Model file for the job. Use its own axes, mm. Face numbers are marked on the shaded views. A direction names the side the tool comes from. Round coordinates to 2 decimals unless told otherwise and drop trailing zeros. Order: outer loops, then holes, each group sorted by start corner. A loop starts at its lowest first (then second) coordinate and runs counter-clockwise, first axis right, second up. Notation, with made-up numbers: M -12,35 L 22,35 A21 cw 22,63 Z; hole C 78.5,23.5 d1. An arc over 180 degrees is marked long. Return JSON: item names as keys, results as strings. Group by question number.
Item 1: Slice it at B-B on y = 0. Write the cut outline in (x, z), then the cut area to 3 significant figures.
Item 2: Which spindle directions (+Z, -Z, +X, -X, +Y, -Y) get a long thin tool onto all of the face, cutting with end or side? Do the marked faces 5 and 6. Say none if no direction does.
Item 3: Slice it at C-C on z = -0.5. Write the cut outline in (x, y).
Item 4: Slice it at D-D on y = 2. Write the cut outline in (x, z), then the cut area to 3 significant figures.
Item 5: Pull direction X, two halves, no side cores. Call the marked faces 1, 2, 3 and 4: pulls with the +X half, pulls with the -X half, needs draft (parallel to the pull), parting line crosses it, or undercut.
Item 6: Slice it at A-A on x = 0. Write the cut outline in (y, z).
Item 7: Pin check, flat tips, straight feed: pin 1 Ø5 at (x, z) = (0, -3) entering from -Y; pin 2 Ø5 at (x, z) = (0, 12) entering from +Y; pin 3 Ø6 at (y, z) = (2, 11.5) entering from -X. Stop position of each tip, or through.
Item 8: Probe line 1 along Z through (x, y) = (0, 2.25); line 2 along X through (y, z) = (-3.25, -3); line 3 along X through (y, z) = (0.75, -3). List the from-to ranges inside material, lowest first.
from build123d import *

# Parameters (mm, degrees)
SKETCH1_R               = 5.5
BOSS_EXTRUDE1_DEPTH     = 9
SKETCH2_R               = 4.5
BOSS_EXTRUDE2_DEPTH     = 6
SKETCH3_R               = 4.5
BOSS_EXTRUDE3_DEPTH     = 6
SKETCH4_R               = 1.5
CUT_EXTRUDE1_DEPTH      = 6.5
CUT_EXTRUDE1_DEPTH_BACK = 6.5


with BuildPart() as part:
    # Sketch1 → Boss-Extrude1 (new body)
    with BuildSketch(Plane.XY):
        Circle(SKETCH1_R)
    extrude(amount=BOSS_EXTRUDE1_DEPTH)

    # Sketch2 → Boss-Extrude2 (add)
    with BuildSketch(Plane.XY.offset(9)):
        Circle(SKETCH2_R)
    extrude(amount=BOSS_EXTRUDE2_DEPTH)

    # Sketch3 → Boss-Extrude3 (add)
    with BuildSketch(Plane(origin=(0, 0, 0), x_dir=(-1, 0, 0), z_dir=(0, 0, -1))):
        Circle(SKETCH3_R)
    extrude(amount=BOSS_EXTRUDE3_DEPTH)

    # Sketch4 → Cut-Extrude1 (cut, two sides)
    with BuildSketch(Plane(origin=(0, 0, 0), x_dir=(1, 0, 0), z_dir=(0, 1, 0))) as cut_extrude1_sk:
        with Locations((0, 3)):
            Circle(SKETCH4_R)
        with Locations((0, -12)):
            Circle(SKETCH4_R)
    extrude(amount=CUT_EXTRUDE1_DEPTH, mode=Mode.SUBTRACT)
    extrude(cut_extrude1_sk.sketch, amount=-CUT_EXTRUDE1_DEPTH_BACK, mode=Mode.SUBTRACT)


solid = part.part
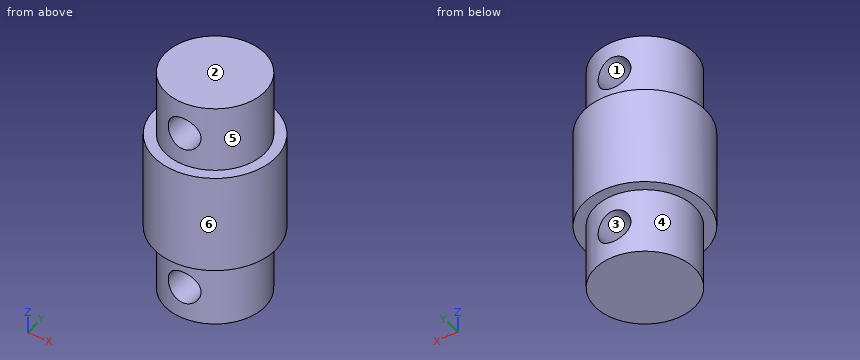
Output values:
{
 "1": {"outline": "M -5.5,0 L -4.5,0 L -4.5,-6 L 4.5,-6 L 4.5,0 L 5.5,0 L 5.5,9 L 4.5,9 L 4.5,15 L -4.5,15 L -4.5,9 L -5.5,9 Z; hole C 0,-3 d3; hole C 0,12 d3", "area": "193 mm²"},
 "2": {"face 5": "+Z", "face 6": "+Z, -Z"},
 "3": {"outline": "C 0,0 d9"},
 "4": {"outline": "M -5.12,0 L -4.03,0 L -4.03,-6 L 4.03,-6 L 4.03,0 L 5.12,0 L 5.12,9 L 4.03,9 L 4.03,15 L -4.03,15 L -4.03,9 L -5.12,9 Z; hole C 0,-3 d3; hole C 0,12 d3", "area": "175 mm²"},
 "5": {"face 1": "undercut", "face 2": "needs draft", "face 3": "undercut", "face 4": "parting line crosses it"},
 "6": {"outline": "M -5.5,0 L -4.5,0 L -4.5,-1.5 L 4.5,-1.5 L 4.5,0 L 5.5,0 L 5.5,9 L 4.5,9 L 4.5,10.5 L -4.5,10.5 L -4.5,9 L -5.5,9 Z; M -4.5,-6 L 4.5,-6 L 4.5,-4.5 L -4.5,-4.5 Z; M -4.5,13.5 L 4.5,13.5 L 4.5,15 L -4.5,15 Z"},
 "7": {"pin 1": "y = -4.5", "pin 2": "y = 4.5", "pin 3": "x = -5.49"},
 "8": {"line 1": "-6 to -4.5, -1.5 to 10.5, 13.5 to 15", "line 2": "-3.11 to -1.5, 1.5 to 3.11", "line 3": "-4.44 to -1.5, 1.5 to 4.44"}
}
